Drawing for the job (mm, zero at the part's lowest x, y, z). Give positions to 0.01 mm unless a question says otherwise; leave off trailing zeros. Write each loop counter-clockwise with the first axis right and the second up, starting at its lowest first coordinate (ties: lowest second). Pieces come first, ordered by that corner, then holes. Notation, with made-up numbers: M -11,11 L 42,11 A37 ccw 42,47 Z; hole C 87,31.5 d11. An arc over 180 degrees is marked long. Use CSV: the item, a comma, the result in double quotes. Start each with the question number.
1. Mould opens along Z. For the marked faces 1 and 2 say: pulls with the +Z half, pulls with the -Z half, needs draft (parallel to the pull), parting line crosses it, or undercut.
2. Drop a flat-ended pin along its axis: pin 1 Ø5.5 at (x, z) = (18.5, 26.5) entering from +Y. Give the stop position or say it passes through.
3. Band-saw the part on D-D, the plane x = 16. List the corners of the cut face in (y, z), then the cut area to 3 significant figures.
4. Band-saw the part on C-C, the plane z = 4. List the corners of the cut face in (x, y).
5. Band-saw the part on B-B, the plane y = 4.25. List the corners of the cut face in (x, z).
6. Band-saw the part on A-A, the plane x = 28. List the corners of the cut face in (y, z), then the cut area to 3 significant figures.
7. Drill centre lines: line 1 along Z through (x, y) = (28, 4.25); line 2 along X through (y, z) = (4.75, 35.5); line 3 along Z through (x, y) = (3, 6.5). Where is each one in solid material? Low to high. Write a range as from..to.
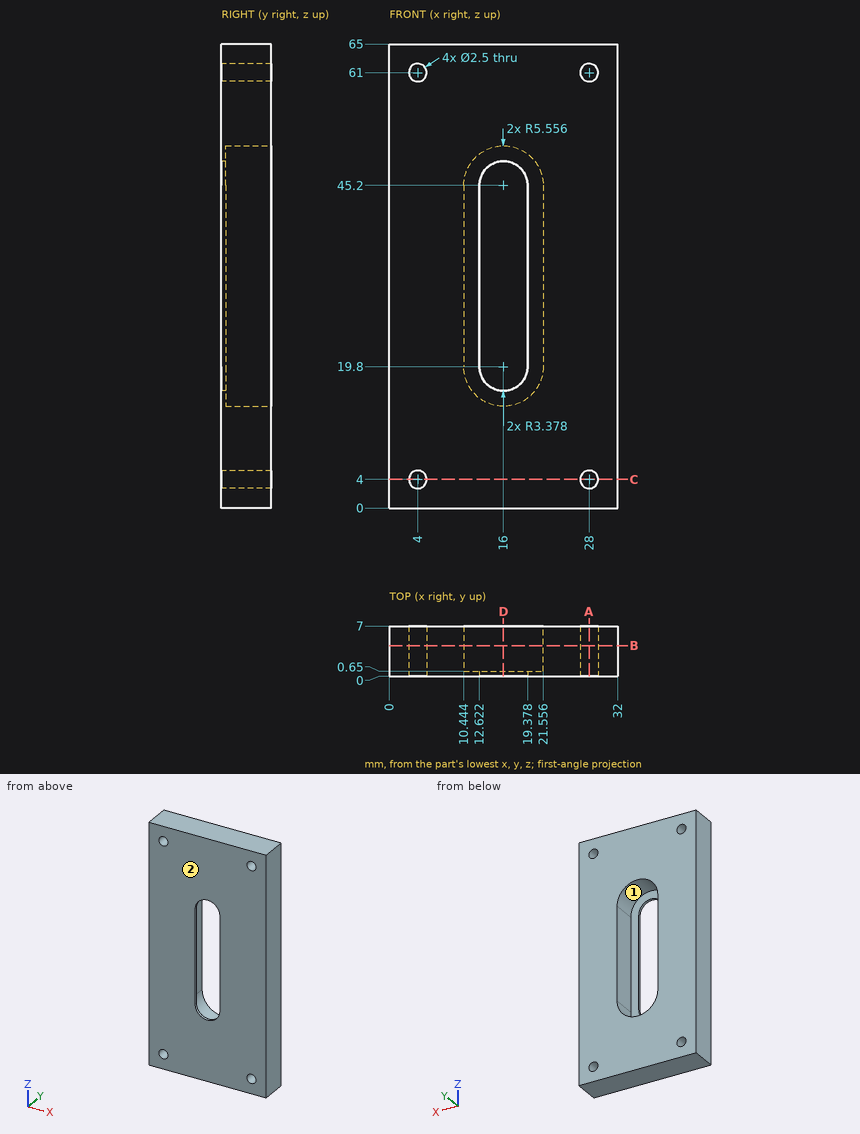
Output:
1,face 1,"undercut"
1,face 2,"needs draft"
2,pin 1,"stops at y = 0.65"
3,outline,"M 0,0 L 7,0 L 7,14.24 L 0.65,14.24 L 0.65,16.42 L 0,16.42 Z; M 0,48.58 L 0.65,48.58 L 0.65,50.76 L 7,50.76 L 7,65 L 0,65 Z"
3,area,"202 mm²"
4,outline,"M 0,0 L 2.75,0 L 2.75,7 L 0,7 Z; M 5.25,0 L 26.75,0 L 26.75,7 L 5.25,7 Z; M 29.25,0 L 32,0 L 32,7 L 29.25,7 Z"
5,outline,"M 0,0 L 32,0 L 32,65 L 0,65 Z; hole C 4,4 d2.5; hole C 4,61 d2.5; hole M 10.44,19.8 A5.56 ccw 21.56,19.8 L 21.56,45.2 A5.56 ccw 10.44,45.2 Z; hole C 28,4 d2.5; hole C 28,61 d2.5"
6,outline,"M 0,0 L 7,0 L 7,2.75 L 0,2.75 Z; M 0,5.25 L 7,5.25 L 7,59.75 L 0,59.75 Z; M 0,62.25 L 7,62.25 L 7,65 L 0,65 Z"
6,area,"420 mm²"
7,line 1,"z = 0..2.75, 5.25..59.75, 62.25..65"
7,line 2,"x = 0..10.44, 21.56..32"
7,line 3,"z = 0..3.25, 4.75..60.25, 61.75..65"
